Part print with two shaded views. Sizes in mm from the minimum x, y, z corner. Coordinates: 2 decimals unless noted, no trailing zeros. Loops run counter-clockwise (first coordinate to the right, second up) from the corner with the lowest first, then second, coordinate; pieces in that order, holes last. Notation, with made-up numbers: (64.25, -14) -> (107.25, -14) arc R25 cw to (107.25, 9) -> close; hole circle Ø2 at (39.5, -2). An arc over 180 degrees is marked (long way). Use one line per item in the form item = value.
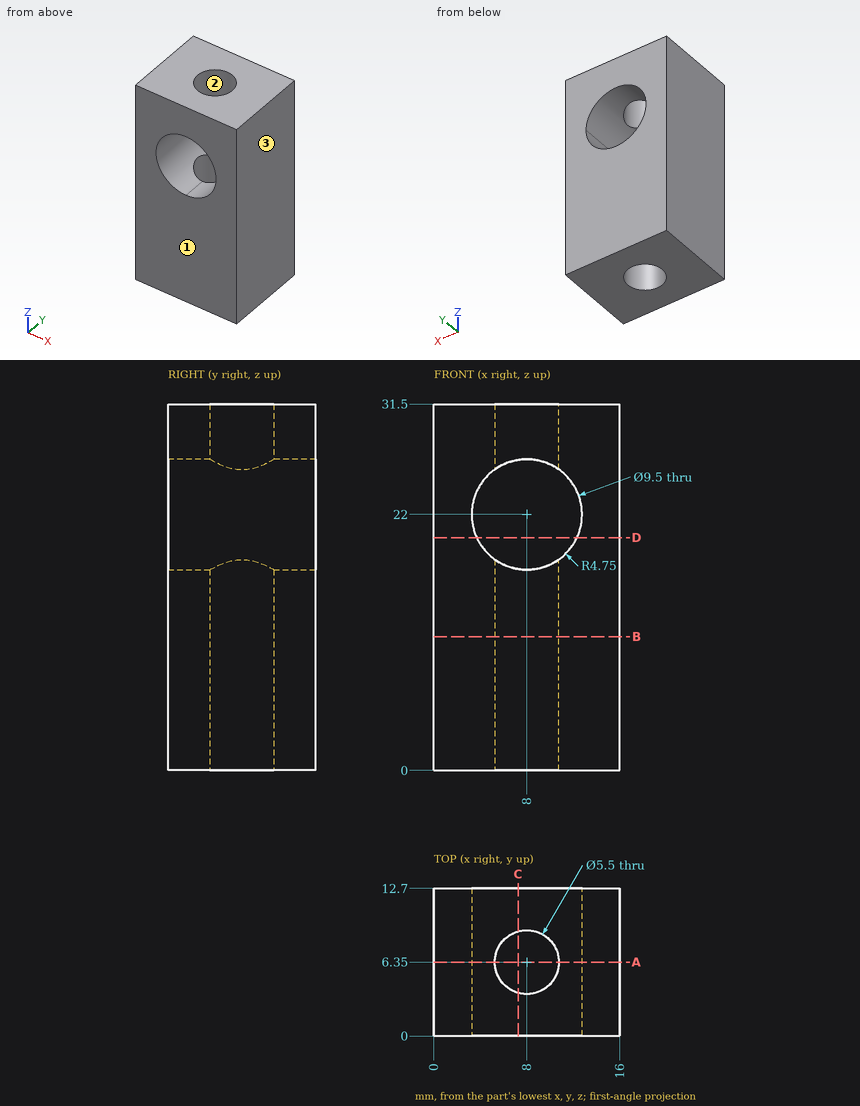
Q1. Pin check, flat tip, straight feed: pin 1 Ø4.5 at (x, y) = (8, 6.35) entering from +Z. Stop position of the tip, or through.
Result:
pin_1 = through
Q2. Band-saw the part on C-C, the plane x = 7.25. Write the cut outline in (y, z), and give its area (3 significant figures).
Result:
outline = (0, 0) -> (3.7, 0) -> (3.7, 17.31) -> (0, 17.31) -> close; (0, 26.69) -> (3.7, 26.69) -> (3.7, 31.5) -> (0, 31.5) -> close; (9, 0) -> (12.7, 0) -> (12.7, 17.31) -> (9, 17.31) -> close; (9, 26.69) -> (12.7, 26.69) -> (12.7, 31.5) -> (9, 31.5) -> close
area = 164 mm2
Q3. Band-saw the part on B-B, the plane z = 11.5. Write the cut outline in (x, y).
Result:
outline = (0, 0) -> (16, 0) -> (16, 12.7) -> (0, 12.7) -> close; hole circle Ø5.5 at (8, 6.35)
Q4. Wall check: line 1 along X through (y, z) = (6.5, 13); line 2 along Y through (x, z) = (8, 12.5); line 3 along Z through (x, y) = (8, 9.75). Give the ranges that are in metal, low to high.
Result:
line_1 = 0 to 5.25, 10.75 to 16
line_2 = 0 to 3.6, 9.1 to 12.7
line_3 = 0 to 17.25, 26.75 to 31.5
Q5. Band-saw the part on A-A, the plane y = 6.35. Write the cut outline in (x, z), and give its area (3 significant figures).
Result:
outline = (0, 0) -> (5.25, 0) -> (5.25, 18.13) arc R4.75 cw to (5.25, 25.87) -> (5.25, 31.5) -> (0, 31.5) -> close; (10.75, 0) -> (16, 0) -> (16, 31.5) -> (10.75, 31.5) -> (10.75, 25.87) arc R4.75 cw to (10.75, 18.13) -> close
area = 309 mm2
Q6. Mould opens along Y. For the marked faces 1, 2 and 3 say: released by +Y, released by -Y, zero draft, split by the parting line, or undercut.
Result:
face_1 = released by -Y
face_2 = undercut
face_3 = zero draft
Q7. Band-saw the part on D-D, the plane z = 20. Write the cut outline in (x, y).
Result:
outline = (0, 0) -> (3.69, 0) -> (3.69, 12.7) -> (0, 12.7) -> close; (12.31, 0) -> (16, 0) -> (16, 12.7) -> (12.31, 12.7) -> close
